Source: CAD feature listing. Evaluate the final solid. Frame: model axes, mm. Round coordinates to 2 decimals unless told otherwise and drop trailing zeros. Order: outer loops, then holes, each group sorted by start corner. A loop starts at its lowest first (then second) coordinate and runs counter-clockwise, first axis right, second up. Notation, with made-up numbers: (31.25, 56) -> (35.25, 56) arc R6 ccw to (35.25, 64) -> close; hole circle Ø9 at (-32, 57). An arc over 180 degrees is marked (long way). Write item = value, one per line. Start each with the question number.
(1) Cut plane A-A on y = 7.25. Return the cut outline in (x, z).
(2) Cut plane C-C on x = -2.5. Return the cut outline in (y, z), then the cut area to 3 significant figures.
(3) Ray query, line 1 (Z direction, x = 1.5, y = 6.5); line 2 (X direction, y = -1.5, z = 185.5). Return the intervals inside material, ascending.
(4) Cut plane D-D on z = 73. Return the cut outline in (x, y).
(5) Contact query for flat-ended pins moving along their axis: pin 1 Ø8 at (x, z) = (1.5, 116) entering from -Y; pin 2 Ø11 at (y, z) = (1, 145) entering from -X; pin 3 Ø2 at (x, z) = (2, 126.5) entering from +Y. Output: stop coordinate, or through.
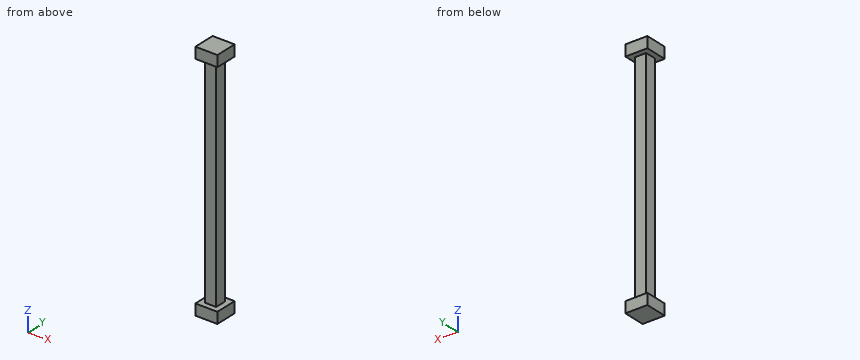
from build123d import *

# Parameters (mm, degrees)
SKETCH_1_W      = 10
SKETCH_1_H      = 10
EXTRUDE_1_DEPTH = 200
SKETCH_2_W      = 20
SKETCH_2_H      = 20
EXTRUDE_2_DEPTH = 10
SKETCH_3_W      = 20
SKETCH_3_H      = 20
EXTRUDE_3_DEPTH = 10


with BuildPart() as part:
    # 草图1 → 凸台-拉伸1 (new body)
    with BuildSketch(Plane.XY):
        Rectangle(SKETCH_1_W, SKETCH_1_H)
    extrude(amount=EXTRUDE_1_DEPTH)

    # 草图2 → 凸台-拉伸2 (add)
    with BuildSketch(Plane.XY.offset(200)):
        Rectangle(SKETCH_2_W, SKETCH_2_H)
    extrude(amount=EXTRUDE_2_DEPTH)

    # 草图3 → 凸台-拉伸3 (add)
    with BuildSketch(Plane(origin=(0, 0, 0), x_dir=(-1, 0, 0), z_dir=(0, 0, -1))):
        Rectangle(SKETCH_3_W, SKETCH_3_H)
    extrude(amount=EXTRUDE_3_DEPTH)


solid = part.part
Evaluation:
q1.outline = (-10, -10) -> (10, -10) -> (10, 0) -> (-10, 0) -> close; (-10, 200) -> (10, 200) -> (10, 210) -> (-10, 210) -> close
q2.outline = (-10, -10) -> (10, -10) -> (10, 0) -> (5, 0) -> (5, 200) -> (10, 200) -> (10, 210) -> (-10, 210) -> (-10, 200) -> (-5, 200) -> (-5, 0) -> (-10, 0) -> close
q2.area = 2,400 mm^2
q3.line_1 = -10 to 0, 200 to 210
q3.line_2 = -5 to 5
q4.outline = (-5, -5) -> (5, -5) -> (5, 5) -> (-5, 5) -> close
q5.pin_1 = -5
q5.pin_2 = -5
q5.pin_3 = 5
